Autodesk Inventor part; units mm, degrees
ref_plane "YZ Plane" through (0, 0, 0) normal (1, 0, 0) x (0, 1, 0)
ref_plane "XZ Plane" through (0, 0, 0) normal (0, 1, 0) x (-1, 0, 0)
ref_plane "XY Plane" through (0, 0, 0) normal (0, 0, 1) x (1, 0, 0)
sketch "Sketch1" plane through (0, 0, 0) normal (0, 1, 0) x (-1, 0, 0)
  line L0 (0, -4.6482) -> (0, -14.4272)
  line L1 (5.9563, -19.05) -> (42.8117, -19.05)
  line L2 (48.768, -14.4272) -> (48.768, -4.6482)
  line L3 (42.8117, 0) -> (5.9563, 0)
  line L4 (0, -14.4272) -> (1.7272, -14.4272)
  line L5 (48.768, -4.6482) -> (47.0408, -4.6482)
  line L6 (48.768, -14.4272) -> (47.0408, -14.4272)
  line L7 (0, -4.6482) -> (1.7272, -4.6482)
  line L8 (24.384, 0) -> (24.384, -19.05) construction
  arc A0 (5.9563, 0) -> (1.7272, -4.6482) centre (5.9563, -4.248) ccw
  arc A1 (1.7272, -14.4272) -> (5.9563, -19.05) centre (5.9586, -14.802) ccw
  arc A2 (47.0408, -4.6482) -> (42.8117, 0) centre (42.8117, -4.248) ccw
  arc A3 (42.8117, -19.05) -> (47.0408, -14.4272) centre (42.8094, -14.802) ccw
  point P0 (0, 0)
  dimension "d1" = 19.05
  dimension "d2" = 48.768
  dimension "d3" = 36.8554
  dimension "d4" = 1.7272
  dimension "d6" = 9.779
  dimension "d8" = 24.384
  dimension "d9" = 4.6482
extrude "Extrusion1" add sketch "Sketch1" along normal blind 25.527
sketch "Sketch2" plane through (0, 25.527, 0) normal (0, 1, 0) x (1, 0, 0)
  line L0 (-46.609, -3.175) -> (-2.159, -3.175)
  line L1 (1.016, 0) -> (1.016, 19.05)
  line L2 (-2.159, 22.225) -> (-46.609, 22.225)
  line L3 (-49.784, 19.05) -> (-49.784, 0)
  line L4 (-5.9563, 19.05) -> (-42.8117, 19.05)
  line L5 (-48.768, 14.4272) -> (-48.768, 4.6482)
  line L6 (-42.8117, 0) -> (-5.9563, 0)
  line L7 (0, 4.6482) -> (0, 14.4272)
  arc A0 (-49.784, 0) -> (-46.609, -3.175) centre (-46.609, 0) ccw
  arc A1 (-46.609, 22.225) -> (-49.784, 19.05) centre (-46.609, 19.05) ccw
  arc A2 (1.016, 19.05) -> (-2.159, 22.225) centre (-2.159, 19.05) ccw
  arc A3 (-2.159, -3.175) -> (1.016, 0) centre (-2.159, 0) ccw
  point P0 (0, 0)
  point P1 (-49.784, -3.175)
  point P2 (1.016, 22.225)
  point P3 (-49.784, 22.225)
  dimension "d13" = 3.175
  dimension "d16" = 1.016
  dimension "d17" = 25.4
  dimension "d18" = 50.8
  dimension "d19" = 3.175
extrude "Extrusion2" add sketch "Sketch2" along normal blind 1.27
sketch "Sketch3" plane through (-42.8117, 0, 0) normal (0, 0, 1) x (1, 0, 0)
  circle A0 centre (5.7277, 9.652) radius 3.175
  circle A1 centre (18.4277, 9.652) radius 3.175
  circle A2 centre (31.1277, 9.652) radius 3.175
  line L0 (-5.9563, 0) -> (-5.9563, 25.527)
  line L1 (0, 25.527) -> (36.8554, 25.527)
  point P0 (42.8117, 0)
  point P1 (43.8277, 25.527)
  point P2 (-6.9723, 25.527)
  dimension "d22" = 12.7
  dimension "d23" = 12.7
  dimension "d25" = 15.875
  dimension "d26" = 6.35
  dimension "d29" = 12.7
extrude "Extrusion3" cut sketch "Sketch3" against normal through all
equation "\"d8\" = 0.5 * d2"
properties part number "ELEV_015_CRSHBLCK1" material "ABS Plastic"
Can you work these out from the model? Positions are in its coordinate system, mm. A direction names the side the tool comes from. Round coordinates to 2 decimals unless told otherwise and drop trailing zeros. Write each loop counter-clockwise with the first axis right and the second up, starting at its lowest first coordinate (ties: lowest second). Pieces come first, ordered by that corner, then holes. Notation, with made-up numbers: (15.25, 2.25) - (51.25, 2.25) arc R23 ccw to (51.25, 16.25) - close; hole circle Ø7 at (6, 50.25). An arc over 180 degrees is marked (long way). Write each question's results on one line, items separated by ' | '. Start each with the question number.
1) Please list where these lines run through material, in increasing order: line 1 (X direction, y = 9.5, z = -15); line 2 (X direction, y = 12.5, z = -18); line 3 (X direction, y = 25, z = -8.5).
2) Which directions (+Z, -Z, +X, -X, +Y, -Y) give clear straight access to the entire face, cutting with the end or side of a thin tool? Please do faces 1 (the flat face through (1.016, 26, -9)), 2 (the flat face through (-25, 15, 0)), 3 (the flat face through (0, 13, -9)), 4 (the flat face through (-24, 15, -19.05)).
3) Suppose I cut it at C-C (y = 7.5). List the corners of the cut face in (x, z) for me.
4) Suppose I cut it at D-D (y = 19.25). List the corners of the cut face in (x, z) for me.
5) Suppose I cut it at B-B (x = -16). List the corners of the cut face in (y, z) for me (3 decimals).
6) We'd pull the mould along Y, two halves only. Please class faces 5 (the cylindrical face through (-35.38, 12.33, -9.39)), 6 (the flat face through (-24, 26, -22.225)), 7 (the flat face through (-24, 0, -9)): released by +Y, released by -Y, zero draft, split by the parting line, or undercut.
7) Suppose I cut it at A-A (z = -15). List the corners of the cut face in (x, y) for me (3 decimals), and give its area (3 significant figures).
8) For pin 1 Ø1.5 at (x, y) = (-37, 14.5) entering from -Z; pin 2 Ø3 at (y, z) = (9.5, -10.5) entering from -X; pin 3 Ø1.4 at (x, y) = (-0.5, 12) entering from +Z; pin 4 Ø5 at (x, y) = (-11.684, 9.652) entering from -Z, each with a flat end and sliding along its axis, tell me the tip position at first contact or that it passes through.
Here are the results:
1) line 1: x = -47.05 to -40.26, -33.91 to -27.56, -21.21 to -14.86, -8.51 to -1.72 | line 2: x = -45.61 to -38.49, -35.68 to -25.79, -22.98 to -13.09, -10.28 to -3.16 | line 3: x = -48.77 to 0
2) face 1: +Z, -Z, +X, +Y, -Y | face 2: +Z, +X, -X, -Y | face 3: +Z, -Z, +X, -Y | face 4: -Z, +X, -X, -Y
3) outline: (-48.77, -14.43) - (-47.04, -14.43) arc R4.25 ccw to (-42.81, -19.05) - (-39.42, -19.05) - (-39.42, 0) - (-42.81, 0) arc R4.25 ccw to (-47.04, -4.65) - (-48.77, -4.65) - close; (-34.75, -19.05) - (-26.72, -19.05) - (-26.72, 0) - (-34.75, 0) - close; (-22.05, -19.05) - (-14.02, -19.05) - (-14.02, 0) - (-22.05, 0) - close; (-9.35, -19.05) - (-5.96, -19.05) arc R4.25 ccw to (-1.73, -14.43) - (0, -14.43) - (0, -4.65) - (-1.73, -4.65) arc R4.25 ccw to (-5.96, 0) - (-9.35, 0) - close
4) outline: (-48.77, -14.43) - (-47.04, -14.43) arc R4.25 ccw to (-42.81, -19.05) - (-5.96, -19.05) arc R4.25 ccw to (-1.73, -14.43) - (0, -14.43) - (0, -4.65) - (-1.73, -4.65) arc R4.25 ccw to (-5.96, 0) - (-42.81, 0) arc R4.25 ccw to (-47.04, -4.65) - (-48.77, -4.65) - close
5) outline: (0, -19.05) - (25.527, -19.05) - (25.527, -22.225) - (26.797, -22.225) - (26.797, 3.175) - (25.527, 3.175) - (25.527, 0) - (0, 0) - close
6) face 5: undercut | face 6: zero draft | face 7: released by -Y
7) outline: (-49.784, 25.527) - (-47.053, 25.527) - (-47.053, 0) - (-1.715, 0) - (-1.715, 25.527) - (1.016, 25.527) - (1.016, 26.797) - (-49.784, 26.797) - close; hole circle Ø6.35 at (-37.084, 9.652); hole circle Ø6.35 at (-24.384, 9.652); hole circle Ø6.35 at (-11.684, 9.652) | area: 1,130 mm2
8) pin 1: stops at z = -19.05 | pin 2: stops at x = -48.77 | pin 3: stops at z = -4.65 | pin 4: passes through
